from build123d import *

# Parameters (mm, degrees)
SKETCH1_R           = 3.25
BOSS_EXTRUDE1_DEPTH = 10
SKETCH2_W           = 29.431964563
SKETCH2_H           = 10
BOSS_EXTRUDE2_DEPTH = 35
SKETCH3_R           = 7.5
CUT_EXTRUDE1_DEPTH  = 35
CHAMFER1_SIZE       = 5


with BuildPart() as part:
    # Sketch1 → Boss-Extrude1 (new body)
    with BuildSketch(Plane(origin=(0, 0, 0), x_dir=(1, 0, 0), z_dir=(0, 1, 0))):
        Polygon((-37.5, -22.474596659), (-37.5, 22.474596659), (-35.5, 24.474596659), (35.5, 24.474596659), (37.5, 22.474596659), (37.5, -22.474596659), (35.5, -24.474596659), (-35.5, -24.474596659), align=None)
        with Locations(Location((-30.5, 17.474596659, 0), (0, 0, 270))):
            Circle(SKETCH1_R, mode=Mode.SUBTRACT)
        with Locations(Location((30.5, 17.474596659, 0), (0, 0, 270))):
            Circle(SKETCH1_R, mode=Mode.SUBTRACT)
        with Locations(Location((30.5, -17.474596659, 0), (0, 0, 90))):
            Circle(SKETCH1_R, mode=Mode.SUBTRACT)
        with Locations(Location((-30.5, -17.474596659, 0), (0, 0, 90))):
            Circle(SKETCH1_R, mode=Mode.SUBTRACT)
    extrude(amount=BOSS_EXTRUDE1_DEPTH)

    # Sketch2 → Boss-Extrude2 (add)
    with BuildSketch(Plane(origin=(0, 10, 0), x_dir=(1, 0, 0), z_dir=(0, 1, 0))):
        with Locations((-2.213221609, -10)):
            Rectangle(SKETCH2_W, SKETCH2_H)
        with Locations((-2.213221609, 10)):
            Rectangle(SKETCH2_W, SKETCH2_H)
    extrude(amount=BOSS_EXTRUDE2_DEPTH)

    # Sketch3 → Cut-Extrude1 (cut)
    with BuildSketch(Plane(origin=(0, 0, -15), x_dir=(-1, 0, 0), z_dir=(0, 0, -1))):
        with Locations((1.786108667, 30)):
            Circle(SKETCH3_R)
    extrude(amount=-CUT_EXTRUDE1_DEPTH, mode=Mode.SUBTRACT)

    # Chamfer1
    chamfer1_edges = [part.edges().sort_by_distance(p)[0] for p in [
        (-16.929203891, 45, -10),
        (12.502760672, 45, -10),
        (12.502760672, 45, 10),
        (-16.929203891, 45, 10),
    ]]
    chamfer(chamfer1_edges, length=CHAMFER1_SIZE)


solid = part.part
Read the model definition and answer for the solid it produces. Units are mm, in the model's axes. A direction names the side the tool comes from. Round coordinates to 2 decimals unless told otherwise and drop trailing zeros. Loops run counter-clockwise (first coordinate to the right, second up) from the corner with the lowest first, then second, coordinate; pieces in that order, holes last. Notation, with made-up numbers: (45, 88) - (96, 88) arc R15 ccw to (96, 111) - close; hole circle Ø1 at (-30.5, 27). An arc over 180 degrees is marked (long way). One line per question, with ' | ' between items. Start each with the question number.
Q1. Section C-C on y = 19.5 is taken. Give the vertices of the cut face in (x, z), plus the area to 3 significant figures.
Q2. Section A-A on y = 30 is taken. Give the vertices of the cut face in (x, z), plus the area to 3 significant figures.
Q3. Section D-D on z = 9 is taken. Give the vertices of the cut face in (x, y), plus the area to 3 significant figures.
Q4. For faces 5 (the flat face through (-6, 23, 15)), 6 (the flat face through (12.503, 25, 10)), 7 (the flat face through (-14.39, 42.54, -9.93)), determine the directions among +Z, -Z, +X, -X, +Y, -Y from which every point of the face is accessible in a straight line to the end or side of a thin tool.
Q5. Section B-B on x = -30.5 is taken. Give the vertices of the cut face in (y, z).
Q6. Find the intervals of material crossed by L1, parallel to Z at x = -7, y = 19; L2, parallel to Z at x = -30, y = 3; L3, parallel to Y at x = 30.5, z = -8, in increasing order.
Q7. For a pull along Z with two mould halves and no side action, classify faces 1 (the flat face through (-6, 23, -15)), 2 (the flat face through (-6, 23, -5)), 3 (the flat face through (-6, 23, 5)), 4 (the flat face through (-16.929, 25, -10)) as +Z half, -Z half, draft (parallel to the pull), parting line (faces both ways), or undercut.
Q8. Flat-ended cylindrical pins translate along their axes: pin 1 (8.5 mm diameter, centred on x = 30.5, z = 17.47, fed in from +Y); pin 2 (9 mm diameter, centred on x = 5, y = 26, fed in from -Z); pin 3 (12 mm diameter, centred on x = -1.79, y = 30, fed in from -Z); pin 4 (2 mm diameter, centred on y = 23, z = -15, fed in from -X). Find the tip coordinate at first contact, or state that the pin passes through.
Established:
1) outline: (-16.93, -15) - (12.5, -15) - (12.5, -5) - (-16.93, -5) - close; (-16.93, 5) - (12.5, 5) - (12.5, 15) - (-16.93, 15) - close | area: 589 mm²
2) outline: (-16.93, -15) - (-9.29, -15) - (-9.29, -5) - (-16.93, -5) - close; (-16.93, 5) - (-9.29, 5) - (-9.29, 15) - (-16.93, 15) - close; (5.71, -15) - (12.5, -15) - (12.5, -5) - (5.71, -5) - close; (5.71, 5) - (12.5, 5) - (12.5, 15) - (5.71, 15) - close | area: 289 mm²
3) outline: (-37.5, 0) - (37.5, 0) - (37.5, 10) - (12.5, 10) - (12.5, 40) - (7.5, 45) - (-11.93, 45) - (-16.93, 40) - (-16.93, 10) - (-37.5, 10) - close; hole circle Ø15 at (-1.79, 30) | area: 1,580 mm²
4) face 5: +Z, +X, -X, +Y | face 6: +Z, -Z, +X, +Y | face 7: +Z, -Z, -X, +Y
5) outline: (0, -24.47) - (10, -24.47) - (10, -20.72) - (0, -20.72) - close; (0, -14.22) - (10, -14.22) - (10, 14.22) - (0, 14.22) - close; (0, 20.72) - (10, 20.72) - (10, 24.47) - (0, 24.47) - close
6) L1: -15 to -5, 5 to 15 | L2: -24.47 to -20.69, -14.26 to 14.26, 20.69 to 24.47 | L3: 0 to 10
7) face 1: -Z half | face 2: undercut | face 3: undercut | face 4: draft
8) pin 1: y = 10 | pin 2: z = -15 | pin 3: through | pin 4: x = -16.93
